Check sheet for the modelled part. Datum: model origin and axes. Units: mm. Give positions to 0.01 mm unless a question says otherwise; leave off trailing zeros. Order: outer loops, then holes, each group sorted by start corner. A loop starts at its lowest first (then second) coordinate and runs counter-clockwise, first axis right, second up. Notation, with made-up numbers: (73.25, 58.25) -> (131.25, 58.25) arc R4 ccw to (131.25, 64.25) -> close; hole circle Ø11 at (-35.75, 36). An arc over 180 degrees is marked (long way). One line per question, with ' | ' between items. Start each with the question number.
from build123d import *

# Parameters (mm, degrees)
CROQUIS1_R              = 100
CROQUIS1_R_2            = 4.025
CROQUIS1_W              = 25.4
CROQUIS1_H              = 25.4
SALIENTE_EXTRUIR1_DEPTH = 2


with BuildPart() as part:
    # Croquis1 → Saliente-Extruir1 (new body)
    with BuildSketch(Plane.XY):
        Circle(CROQUIS1_R)
        with Locations((0, 85)):
            Circle(CROQUIS1_R_2, mode=Mode.SUBTRACT)
        with Locations((60.104076401, 60.104076401)):
            Circle(CROQUIS1_R_2, mode=Mode.SUBTRACT)
        with Locations((85, 0)):
            Circle(CROQUIS1_R_2, mode=Mode.SUBTRACT)
        with Locations((60.104076401, -60.104076401)):
            Circle(CROQUIS1_R_2, mode=Mode.SUBTRACT)
        with Locations((0, -85)):
            Circle(CROQUIS1_R_2, mode=Mode.SUBTRACT)
        with Locations((-60.104076401, -60.104076401)):
            Circle(CROQUIS1_R_2, mode=Mode.SUBTRACT)
        with Locations((-85, 0)):
            Circle(CROQUIS1_R_2, mode=Mode.SUBTRACT)
        with Locations((-60.104076401, 60.104076401)):
            Circle(CROQUIS1_R_2, mode=Mode.SUBTRACT)
        Rectangle(CROQUIS1_W, CROQUIS1_H, mode=Mode.SUBTRACT)
    extrude(amount=SALIENTE_EXTRUIR1_DEPTH)


solid = part.part
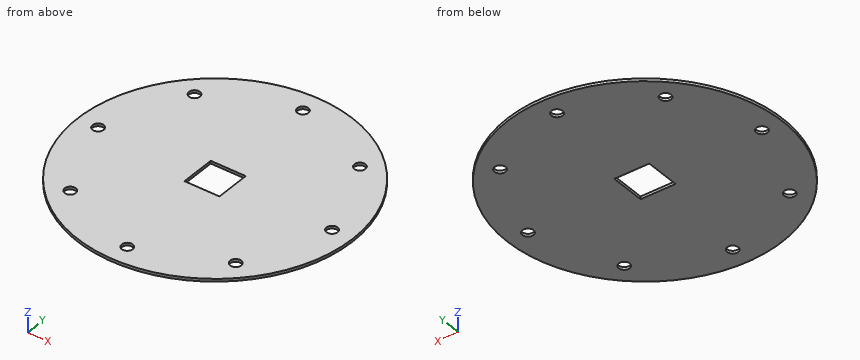
1. Cross-section at A-A on x = 0. Record the boundary of the cut face in (y, z) (3 decimals), and give its area (3 significant figures).
2. Scan lines: probe 1 along X at (y, z) = (58, 0.8); probe 2 along Y at (x, z) = (1, 1.8) (3 decimals); probe 3 along Y at (x, z) = (-87, 1.1). Record each from-to range of solid material in increasing order.
3. Cross-section at D-D on z = 1.65. Give the number of separate pieces and of enclosed holes in the cut face, and give its area (3 significant figures).
4. Go/stop test with flat-tipped pins: pin 1 (10.5 mm diameter, centred on x = 0, y = 85, fed in from +Z); pin 2 (0.6 mm diameter, centred on x = -4.5, z = 0.5, fed in from -Y); pin 3 (0.6 mm diameter, centred on y = -4.5, z = 1, fed in from +X); pin 4 (1 mm diameter, centred on y = 5, z = 0.5, fed in from -X). Record where each tip stops, or that it passes through.
5. Cross-section at C-C on x = -60. Record the boundary of the cut face in (y, z).
Response values:
1) outline: (-100, 0) -> (-89.025, 0) -> (-89.025, 2) -> (-100, 2) -> close; (-80.975, 0) -> (-12.7, 0) -> (-12.7, 2) -> (-80.975, 2) -> close; (12.7, 0) -> (80.975, 0) -> (80.975, 2) -> (12.7, 2) -> close; (89.025, 0) -> (100, 0) -> (100, 2) -> (89.025, 2) -> close | area: 317 mm²
2) probe 1: x = -81.46 to -63.54, -56.67 to 56.67, 63.54 to 81.46 | probe 2: y = -99.995 to -88.899, -81.101 to -12.7, 12.7 to 81.101, 88.899 to 99.995 | probe 3: y = -49.31 to -3.49, 3.49 to 49.31
3) separate pieces: 1 | enclosed holes: 9 | area: 30,400 mm²
4) pin 1: stops at z = 2 | pin 2: stops at y = -99.91 | pin 3: stops at x = 99.91 | pin 4: stops at x = -99.9
5) outline: (-80, 0) -> (-64.13, 0) -> (-64.13, 2) -> (-80, 2) -> close; (-56.08, 0) -> (56.08, 0) -> (56.08, 2) -> (-56.08, 2) -> close; (64.13, 0) -> (80, 0) -> (80, 2) -> (64.13, 2) -> close
